Can you work these out from the model? Positions are in its coordinate system, mm. A direction names the side the tool comes from. Give positions to 0.01 mm unless a question says otherwise; leave off trailing zeros. Loops run counter-clockwise (first coordinate to the right, second up) from the corner with the lowest first, then second, coordinate; pieces in that order, holes last. Notation, with made-up numbers: (-34, 79.25) - (13, 79.25) arc R18 ccw to (13, 108.25) - close; hole circle Ø4 at (20, 81). An arc over 180 degrees is marked (long way). Write item = value, one per line.
from build123d import *

# Parameters (mm, degrees)
F0_W     = 50
F0_H     = 40
F1_DEPTH = 2
F3_DEPTH = 12.5
F4_R     = 25
F5_DEPTH = 7.5
F6_R     = 4
F7_R     = 4.99999


# Not quite as in the source:
# - a fillet or chamfer is up to 0.001 mm smaller than in the source, because OpenCascade refuses the exact size


with BuildPart() as f1:
    # F0 (on Top) → F1 (new body)
    with BuildSketch(Plane.XY):
        Rectangle(F0_W, F0_H)
    extrude(amount=F1_DEPTH)

    # F2 (on Front) → F3 (join, symmetric)
    with BuildSketch(Plane.XZ):
        with BuildLine():
            Line((12.5, 0), (-12.5, 0))
            Line((-12.5, 0), (-12.5, -30.5279912201))
            ThreePointArc((-12.5, -30.5279912201), (-11.7069556163, -34.43080665), (-9.4536063441, -37.7146009084))
            Line((-9.4536063441, -37.7146009084), (6.3529476633, -53.0086768346))
            ThreePointArc((6.3529476633, -53.0086768346), (22.3177107814, -52.745608492), (22.0546424389, -36.7808453739))
            Line((22.0546424389, -36.7808453739), (14.4186308033, -20.6281161927))
            ThreePointArc((14.4186308033, -20.6281161927), (12.9855517125, -16.4605806119), (12.5, -12.0803628053))
            Line((12.5, -12.0803628053), (12.5, 0))
        make_face()
    extrude(amount=F3_DEPTH, both=True)

    # F4 (on Front) → F5 (join, symmetric)
    with BuildSketch(Plane.XZ):
        with Locations((13.390565291, -43)):
            Circle(F4_R)
    extrude(amount=F5_DEPTH, both=True)

    # F6
    f6_edges = [f1.edges().sort_by_distance(p)[0] for p in [
        (28.500684, -7.5, -62.916935),
        (28.500684, 7.5, -62.916935),
    ]]
    fillet(f6_edges, radius=F6_R)

    # F7 (radius 5 in the source; OpenCascade refuses exactly that, so slightly less here)
    f7_edges = [f1.edges().sort_by_distance(p)[0] for p in [
        (12.5, -12.5, -6.040181),
        (-12.5, -12.5, -15.263996),
        (-12.5, 12.5, -15.263996),
        (12.5, 12.5, -6.040181),
    ]]
    fillet(f7_edges, radius=F7_R)


solid = f1.part
Q1. I need wall thicknesses on L1, parallel to X at y = 7, z = -7.5; L2, parallel to Z at x = -12.5, y = -12.5. Which ranges of each line are inside material? Lowest first, please.
Output:
L1 = -12.5 to 12.5
L2 = 0 to 2
Q2. Imagine slicing it at A-A, the plane y = -5.5. Write out the boundary of the cut face in (x, z), then the cut area to 3 significant figures.
Output:
outline = (-25, 0) - (-12.5, 0) - (-12.5, -30.53) arc R10 ccw to (-10.28, -36.81) arc R24.46 ccw (long way) to (13.57, -18.54) arc R20 cw to (12.5, -12.08) - (12.5, 0) - (25, 0) - (25, 2) - (-25, 2) - close
area = 2,590 mm2
Q3. We'd pull the mould along Z, two halves only. Please class faces 6 (the flat face through (18, -7.5, -57)), 7 (the flat face through (0, -20, 1)), 8 (the flat face through (0, 0, 2)): released by +Z, released by -Z, zero draft, split by the parting line, or undercut.
Output:
face_6 = undercut
face_7 = zero draft
face_8 = released by +Z
Q4. Which directions (+Z, -Z, +X, -X, +Y, -Y) give clear straight access to the entire face, cutting with the end or side of a thin tool? Please do faces 1 (the flat face through (3, -12.5, -25)), 2 (the flat face through (-12.5, 0, -15)), 3 (the flat face through (-9.2, 7.27, -37.96)), 4 (the flat face through (-9.2, -7.27, -37.96)), 5 (the cylindrical face through (11, 11.07, -5.96)).
Output:
face_1 = -Z, +X, -X, -Y
face_2 = -Z, -X, +Y, -Y
face_3 = -X, +Y
face_4 = -X, -Y
face_5 = +X, +Y
Q5. Imagine slicing it at D-D, the plane y = 4.5. Write out the boundary of the cut face in (x, z), then the cut area to 3 significant figures.
Output:
outline = (-25, 0) - (-12.5, 0) - (-12.5, -30.53) arc R10 ccw to (-10.59, -36.4) arc R24.87 ccw (long way) to (13.44, -18.13) arc R20 cw to (12.5, -12.08) - (12.5, 0) - (25, 0) - (25, 2) - (-25, 2) - close
area = 2,640 mm2
Q6. Imagine slicing it at C-C, the plane x = -20. Write out the boundary of the cut face in (y, z), then the cut area to 3 significant figures.
Output:
outline = (-20, 0) - (20, 0) - (20, 2) - (-20, 2) - close
area = 80.0 mm2
Q7. Imagine slicing it at B-B, the plane z = -7.5. Write out the boundary of the cut face in (x, y).
Output:
outline = (-12.5, -7.5) arc R5 ccw to (-7.5, -12.5) - (7.5, -12.5) arc R5 ccw to (12.5, -7.5) - (12.5, 7.5) arc R5 ccw to (7.5, 12.5) - (-7.5, 12.5) arc R5 ccw to (-12.5, 7.5) - close
Q8. For pin 1 (0.6 mm diameter, centred on y = -6, z = 0.5, fed in from +X); pin 2 (8.5 mm diameter, centred on x = 6.5, z = -21, fed in from -Y); pin 3 (3.5 mm diameter, centred on y = 0, z = -5.5, fed in from +X), each with a flat end and sliding along its axis, tell me the tip position at first contact or that it passes through.
Output:
pin_1 = 25
pin_2 = -12.5
pin_3 = 12.5
